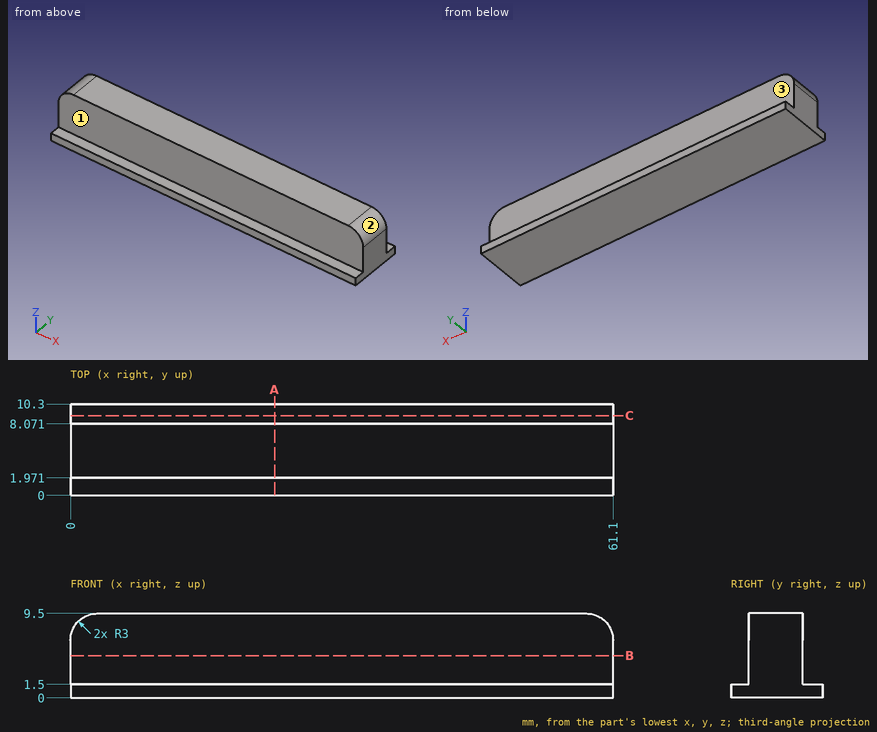
Here's the drawing with two shaded views (mm, measured from the low corner). I have some questions. A direction names the side the tool comes from. Coordinates: 2 decimals unless noted, no trailing zeros. Order: outer loops, then holes, each group sorted by start corner. A loop starts at its lowest first (then second) coordinate and runs counter-clockwise, first axis right, second up.
Q1. Suppose I cut it at A-A on x = 23. Please give me the cut outline in (y, z).
Q2. Will these pins go through, and if not, where does the flat tip stop? pin 1 (1.1 mm diameter, centred on x = 42, y = 9, fed in from +Z); pin 2 (6 mm diameter, centred on x = 51, y = 1, fed in from +Z); pin 3 (3 mm diameter, centred on x = 30, z = 6.5, fed in from -Y).
Q3. Suppose I cut it at C-C on y = 9. Please give me the cut outline in (x, z).
Q4. Which directions (+Z, -Z, +X, -X, +Y, -Y) give clear straight access to the entire face, cutting with the end or side of a thin tool? Please do the marked faces 1, 2 and 3.
Q5. Please list where these lines run through material, in increasing order: L1, parallel to Y at x = 22, z = 5.5; L2, parallel to Z at x = 32, y = 1.75; L3, parallel to X at y = 4.25, z = 8.75 (1 decimal).
Q6. Suppose I cut it at B-B on z = 4.75. Please give me the cut outline in (x, y), and give its area (3 significant figures).
Answer:
1. outline: (0, 0) - (10.3, 0) - (10.3, 1.5) - (8.07, 1.5) - (8.07, 9.5) - (1.97, 9.5) - (1.97, 1.5) - (0, 1.5) - close
2. pin 1: stops at z = 1.5
2. pin 2: stops at z = 9.5
2. pin 3: stops at y = 1.97
3. outline: (0, 0) - (61.1, 0) - (61.1, 1.5) - (0, 1.5) - close
4. face 1: +Z, +X, -X, -Y
4. face 2: +Z, +X, +Y, -Y
4. face 3: +Z, +X, -X, +Y
5. L1: y = 1.97 to 8.07
5. L2: z = 0 to 1.5
5. L3: x = 1 to 60.1
6. outline: (0, 1.97) - (61.1, 1.97) - (61.1, 8.07) - (0, 8.07) - close
6. area: 373 mm2
